The model under review builds one solid part; all positions refer to its coordinate system, in mm. Coordinates: 2 decimals unless noted, no trailing zeros. Loops run counter-clockwise (first coordinate to the right, second up) from the corner with the lowest first, then second, coordinate; pieces in that order, holes last. Notation, with made-up numbers: M -12,67 L 18,67 A21 cw 18,81 Z; hole C 73,27.5 d1. An arc over 180 degrees is marked long. Return JSON: item names as keys, results as strings.
Autodesk Inventor part; units mm, degrees
ref_plane "YZ Plane" through (0, 0, 0) normal (1, 0, 0) x (0, 1, 0)
ref_plane "XZ Plane" through (0, 0, 0) normal (0, 1, 0) x (-1, 0, 0)
ref_plane "XY Plane" through (0, 0, 0) normal (0, 0, 1) x (1, 0, 0)
sketch "ThunderHex" plane through (0, 0, 0) normal (0, 0, 1) x (1, 0, 0)
  line L0 (0, 0) -> (5.1191, 0)
  line L1 (6.801, -0.9711) -> (9.3605, -5.4043)
  arc A0 (0, 0) -> (-1.682, -0.9711) centre (2.5595, -6.3754) ccw
  arc A1 (9.3605, -7.3465) -> (9.3605, -5.4043) centre (2.5595, -6.3754) ccw
  circle A2 centre (2.5595, -6.3754) radius 2.55
  line L2 (-4.2415, -5.4043) -> (-1.682, -0.9711)
  arc A3 (-4.2415, -5.4043) -> (-4.2415, -7.3465) centre (2.5595, -6.3754) ccw
  line L3 (-1.682, -11.7797) -> (-4.2415, -7.3465)
  arc A4 (-1.682, -11.7797) -> (0, -12.7508) centre (2.5595, -6.3754) ccw
  line L4 (5.1191, -12.7508) -> (0, -12.7508)
  arc A5 (5.1191, -12.7508) -> (6.801, -11.7797) centre (2.5595, -6.3754) ccw
  line L5 (9.3605, -7.3465) -> (6.801, -11.7797)
  arc A6 (6.801, -0.9711) -> (5.1191, 0) centre (2.5595, -6.3754) ccw
  point P0 (2.5595, -6.3754)
sketch "Sketch1" plane through (0, 0, 0) normal (0, 0, 1) x (1, 0, 0)
  line L0 (-2.5595, 6.3754) -> (2.5595, 6.3754)
  line L1 (4.2415, 5.4043) -> (6.801, 0.9711)
  arc A0 (-2.5595, 6.3754) -> (-4.2415, 5.4043) centre (0, 0) ccw
  arc A1 (6.801, -0.9711) -> (6.801, 0.9711) centre (0, 0) ccw
  circle A2 centre (0, 0) radius 2.55
  line L2 (-6.801, 0.9711) -> (-4.2415, 5.4043)
  arc A3 (-6.801, 0.9711) -> (-6.801, -0.9711) centre (0, 0) ccw
  line L3 (-4.2415, -5.4043) -> (-6.801, -0.9711)
  arc A4 (-4.2415, -5.4043) -> (-2.5595, -6.3754) centre (0, 0) ccw
  line L4 (2.5595, -6.3754) -> (-2.5595, -6.3754)
  arc A5 (2.5595, -6.3754) -> (4.2415, -5.4043) centre (0, 0) ccw
  line L5 (6.801, -0.9711) -> (4.2415, -5.4043)
  arc A6 (4.2415, 5.4043) -> (2.5595, 6.3754) centre (0, 0) ccw
extrude "Extrusion1" add sketch "Sketch1" along normal mid plane 304.8
properties part number "ThunderHex" material "Aluminum 6061"
1. Add section A-A on x = 0. Give the boundary of the cut face in (y, z).
Check values:
{"outline": "M -6.38,-152.4 L -2.55,-152.4 L -2.55,152.4 L -6.38,152.4 Z; M 2.55,-152.4 L 6.38,-152.4 L 6.38,152.4 L 2.55,152.4 Z"}
2. The part is to be moulded in two halves that separate along X. For faces 1 (the face through (0, 6.375, -2)), 2 (the face through (1.18, 2.26, -2.13)), say which applies: released by +X, released by -X, zero draft, split by the parting line, or undercut.
Check values:
{"face 1": "zero draft", "face 2": "undercut"}
3. To check wall thickness, follow line 1 (Y direction, x = 0, z = 34.5); line 2 (X direction, y = 0.25, z = 64.5); line 3 (Y direction, x = -1, z = 119). State the ranges of each line that lie inside material, in increasing order.
Check values:
{"line 1": "-6.38 to -2.55, 2.55 to 6.38", "line 2": "-6.87 to -2.54, 2.54 to 6.87", "line 3": "-6.38 to -2.35, 2.35 to 6.38"}
4. Insertion check: pin 1 Ø6 at (y, z) = (0.5, -39.5) entering from +X; pin 2 Ø5 at (y, z) = (-4.5, 49.5) entering from -X. Each pin has a flat end and moves straight along its axis. Give the tip position at first contact, or say it passes through.
Check values:
{"pin 1": "x = 6.87", "pin 2": "x = -6.21"}
5. Add section B-B on z = 43.5. Give the boundary of the cut face in (x, y), plus the area to 3 significant figures.
Check values:
{"outline": "M -6.8,-0.97 L -4.24,-5.4 A6.87 ccw -2.56,-6.38 L 2.56,-6.38 A6.87 ccw 4.24,-5.4 L 6.8,-0.97 A6.87 ccw 6.8,0.97 L 4.24,5.4 A6.87 ccw 2.56,6.38 L -2.56,6.38 A6.87 ccw -4.24,5.4 L -6.8,0.97 A6.87 ccw Z; hole C 0,0 d5.1", "area": "118 mm²"}
